Geometry: final body of the model. Coordinates: model frame, mm. A direction names the side the tool comes from. Coordinates: 2 decimals unless noted, no trailing zeros. Write each loop counter-clockwise with the first axis right and the second up, starting at its lowest first coordinate (ties: lowest second). Pieces come first, ordered by that corner, then holes.
from build123d import *

# Parameters (mm, degrees)
BOSS_EXTRUDE1_DEPTH = 100
CUT_EXTRUDE1_DEPTH  = 126.95237195067031
FILLET1_R           = 5
BOSS_EXTRUDE2_START = 40.5
BOSS_EXTRUDE2_DEPTH = 40.5
FILLET2_R           = 11
FILLET3_R           = 5
BOSS_EXTRUDE4_DEPTH = 10
FILLET5_R           = 1
FILLET6_R           = 5
SKETCH8_R           = 7.5
CUT_EXTRUDE2_DEPTH  = 131.85870255202755
SKETCH9_R           = 1.2499999999993074
SKETCH9_R_2         = 1.2499999999993041
SKETCH9_R_3         = 1.2499999999993108
CUT_EXTRUDE3_DEPTH  = 131.85870255202755
SKETCH10_R          = 2.999999999999271
SKETCH10_R_2        = 2.9999999999993827
SKETCH10_R_3        = 2.9999999999993676
SKETCH10_R_4        = 2.9999999999984848
CUT_EXTRUDE4_DEPTH  = 5


with BuildPart() as part:
    # Sketch1 → Boss-Extrude1 (new body)
    with BuildSketch(Plane(origin=(0, 0, 0), x_dir=(1, 0, 0), z_dir=(0, 1, 0))):
        Polygon((-29.000000000000004, -50), (-29.000000000000004, 50), (28.999999999999996, 50.00000000000001), (28.999999999999996, -50), (22.5, -50), (22.49999999999999, 20.000000000000004), (-18.000000000000007, 20.000000000000004), (-18.000000000000007, -50), align=None)
    extrude(amount=BOSS_EXTRUDE1_DEPTH)

    # Sketch5 → Cut-Extrude1 (cut, through all)
    with BuildSketch(Plane(origin=(28.999999999999996, 0, 0), x_dir=(0, 0, -1), z_dir=(1, 0, 0))):
        with BuildLine():
            Line((50.00000000000001, 94), (15.000000000000007, 94))
            Line((15.000000000000007, 94), (-15.988977704079698, 68.21854812358211))
            ThreePointArc((-15.988977704079698, 68.21854812358211), (-24.331609312743236, 43.25780632057522), (-5.709440185764556, 24.660684217398867))
            Line((-5.709440185764556, 24.660684217398867), (44.000000000000014, 12.999999999999998))
            Line((44.000000000000014, 12.999999999999998), (50.00000000000001, 12.999999999999998))
            Line((50.00000000000001, 12.999999999999998), (50.00000000000001, 94))
        make_face()
        with BuildLine():
            Line((12.83046096501491, 100), (-19.82633235305885, 72.8309996732418))
            ThreePointArc((-19.82633235305885, 72.8309996732418), (-30.160384185664846, 41.83402304126666), (-6.988314668956372, 18.797956061093338))
            Line((-6.988314668956372, 18.797956061093338), (44, 6.999999999999997))
            Line((44, 6.999999999999997), (49.99999999999999, 6.999999999999992))
            Line((49.99999999999999, 6.999999999999992), (49.99999999999999, 0))
            Line((49.99999999999999, 0), (-50.00000000000001, 0))
            Line((-50.00000000000001, 0), (-50.00000000000001, 100))
            Line((-50.00000000000001, 100), (12.83046096501491, 100))
        make_face()
    extrude(amount=-CUT_EXTRUDE1_DEPTH, mode=Mode.SUBTRACT)

    # Fillet1
    fillet1_edges = [part.edges().sort_by_distance(p)[0] for p in [
        (-23.500000000000004, 94, -15.000000000000007),
        (25.749999999999993, 94, -15.000000000000007),
    ]]
    fillet(fillet1_edges, radius=FILLET1_R)

    # Sketch6 → Boss-Extrude2 (add)
    with BuildSketch(Plane(origin=(-18.000000000000007, 0, 0), x_dir=(1e-16, 0, -1), z_dir=(1, 0, 1e-16)).offset(BOSS_EXTRUDE2_START)):
        with BuildLine():
            Line((19.999999999999996, 12.553251706878484), (-6.988314668956373, 18.79795606109335))
            ThreePointArc((-6.988314668956373, 18.79795606109335), (-27.865951255157718, 35.417336025463435), (-28.095541398136127, 62.1011661139617))
            Line((-28.095541398136127, 62.1011661139617), (-22.657694675916233, 59.56545654351749))
            ThreePointArc((-22.657694675916233, 59.56545654351749), (-22.489094420401646, 38.08026409887772), (-5.709440185764564, 24.66068421739888))
            Line((-5.709440185764564, 24.66068421739888), (19.999999999999993, 18.62984455611945))
            Line((19.999999999999993, 18.62984455611945), (19.999999999999996, 12.553251706878484))
        make_face()
    extrude(amount=-BOSS_EXTRUDE2_DEPTH)

    # Fillet2
    fillet2_edges = [part.edges().sort_by_distance(p)[0] for p in [
        (25.749999999999993, 100, -12.83046096501491),
        (-23.500000000000004, 100, -12.83046096501491),
    ]]
    fillet(fillet2_edges, radius=FILLET2_R)

    # Fillet3
    fillet3_edges = [part.edges().sort_by_distance(p)[0] for p in [
        (22.49999999999999, 60.8333113287396, 25.376618037026184),
        (-18.00000000000001, 60.8333113287396, 25.37661803702618),
        (22.49999999999999, 97, -20.000000000000004),
        (-18.000000000000007, 97, -20.000000000000004),
    ]]
    fillet(fillet3_edges, radius=FILLET3_R)

    # Sketch7 → Boss-Extrude4 (add)
    with BuildSketch(Plane(origin=(28.999999999999996, 0, 0), x_dir=(0, 0, -1), z_dir=(1, 0, 0))):
        with BuildLine():
            Line((50.00000000000001, 100), (16.807949195820918, 100))
            ThreePointArc((16.807949195820918, 100), (13.067479500591284, 99.34450996708247), (9.772799006025844, 97.45616117437613))
            Line((9.772799006025844, 97.45616117437613), (-19.82633235305885, 72.8309996732418))
            ThreePointArc((-19.82633235305885, 72.8309996732418), (-30.160384185664846, 41.83402304126666), (-6.9883146689563755, 18.797956061093355))
            Line((-6.9883146689563755, 18.797956061093355), (44, 6.999999999999997))
            Line((44, 6.999999999999997), (49.99999999999999, 6.999999999999992))
            Line((49.99999999999999, 6.999999999999992), (50.00000000000001, 100))
        make_face()
    extrude(amount=BOSS_EXTRUDE4_DEPTH)

    # Fillet5
    fillet5_edges = [part.edges().sort_by_distance(p)[0] for p in [
        (22.49999999999999, 99.00083975111619, -12.227206431541916),
        (-18.000000000000007, 85.14358042380897, 5.026766673516516),
        (22.499999999999993, 69.84794587448418, 22.942605623916762),
        (2.2499999999999893, 62.10116611396171, 28.095541398136127),
        (-18.000000000000007, 99.00083975111619, -12.227206431541916),
        (2.2499999999999893, 100, -20.000000000000004),
        (21.042619780265184, 63.42008867833863, 27.44195770208064),
        (-16.542619780265202, 63.42008867833864, 27.441957702080636),
        (20.324911858881205, 100, -19.12551487569155),
        (22.415270684599754, 99.96382489332538, -15.916577372895661),
        (-17.91527069193968, 99.96382489235059, -15.916577374222168),
        (-15.824911858881226, 100, -19.125514875691554),
        (-18.000000000000004, 69.84794587448418, 22.942605623916755),
        (22.49999999999999, 85.14358042380897, 5.026766673516505),
    ]]
    fillet(fillet5_edges, radius=FILLET5_R)

    # Fillet6
    fillet6_edges = [part.edges().sort_by_distance(p)[0] for p in [
        (39, 12.898978030546676, -18.50584266552181),
        (39, 41.834023041266654, 30.16038418566485),
        (39, 85.14358042380897, 5.026766673516503),
        (39, 99.34450996708247, -13.067479500591286),
        (39, 100, -33.40397459791046),
    ]]
    fillet(fillet6_edges, radius=FILLET6_R)

    # Sketch8 → Cut-Extrude2 (cut, through all)
    with BuildSketch(Plane(origin=(39, 0, 0), x_dir=(0, 0, -1), z_dir=(1, 0, 0))):
        with Locations((-6.94e-15, 49)):
            Circle(SKETCH8_R)
    extrude(amount=-CUT_EXTRUDE2_DEPTH, mode=Mode.SUBTRACT)

    # Sketch9 → Cut-Extrude3 (cut, through all)
    with BuildSketch(Plane(origin=(39, 0, 0), x_dir=(0, 0, -1), z_dir=(1, 0, 0))):
        with Locations((40.00000000000071, 19.744580488536943)):
            Circle(SKETCH9_R)
        with Locations((6.9389e-13, 29.000000000001137)):
            Circle(SKETCH9_R_2)
        with Locations((-19.999999999998934, 49.000000000000405)):
            Circle(SKETCH9_R_2)
        with Locations((16.807949195821617, 89.00000000000007)):
            Circle(SKETCH9_R_3)
    extrude(amount=-CUT_EXTRUDE3_DEPTH, mode=Mode.SUBTRACT)

    # Sketch10 → Cut-Extrude4 (cut)
    with BuildSketch(Plane(origin=(39, 0, 0), x_dir=(0, 0, -1), z_dir=(1, 0, 0))):
        with Locations((16.807949195821624, 89.00000000000007)):
            Circle(SKETCH10_R)
        with Locations((-19.999999999998906, 49.000000000000405)):
            Circle(SKETCH10_R_2)
        with Locations((-1.388e-14, 29.000000000001066)):
            Circle(SKETCH10_R_3)
        with Locations((40.000000000000725, 19.744580488536943)):
            Circle(SKETCH10_R_4)
    extrude(amount=-CUT_EXTRUDE4_DEPTH, mode=Mode.SUBTRACT)


solid = part.part
Item 1: Set-up query: faces 5 (the flat face through (0, 13, -47)), 6 (the cylindrical face through (-16.57, 61.86, 24.03)), 7 (the cylindrical face through (36.53, 91.53, -18.42)). Return all of +Z, -Z, +X, -X, +Y, -Y with unobstructed straight access to the full face (end or side cutting, diameter ignored); none if empty.
Derived:
face 5: -Z, -X
face 6: -Z, +Y
face 7: +X
Item 2: Material intervals for probe 1 along X at (y, z) = (78, 6.5); probe 2 along Z at (x, y) = (31.5, 48); probe 3 along X at (y, z) = (50.5, 23), sorted ascending.
Derived:
probe 1: x = -29 to -18, 22.5 to 38.98
probe 2: z = -50 to -7.43, 7.43 to 19.25, 20.75 to 30.98
probe 3: x = 29 to 39
Item 3: Section B-B, the plane y = 49. Output: boundary loops of the cut face in (x, z).
Derived:
outline: (-29, 25) - (29, 25) - (29, 21.25) - (34, 21.25) - (34, 23) - (39, 23) - (39, 26) arc R5 ccw to (34, 31) - (-29, 31) - close; (29, -50) - (39, -50) - (39, -7.5) - (29, -7.5) - close; (29, 7.5) - (39, 7.5) - (39, 17) - (34, 17) - (34, 18.75) - (29, 18.75) - close
Item 4: Pull-direction query (Y, two-part tool) for faces 1 (the cylindrical face through (-18.285, 84.74, 5.042)), 2 (the flat face through (34, 18, -40)), 3 (the flat face through (2.06, 12.98, -18.15)), 4 (the cylindrical face through (-23.4, 93.7, -15.1)); classes: released by +Y, released by -Y, zero draft, split by the parting line, or undercut.
Derived:
face 1: released by +Y
face 2: undercut
face 3: released by -Y
face 4: undercut
Item 5: Pin query (flat end, axial travel): pin 1 (5 mm diameter, centred on y = 49, z = 20, fed in from +X); pin 2 (4 mm diameter, centred on x = 12.5, z = 8, fed in from +Y); pin 3 (10 mm diameter, centred on x = -21.5, y = 21, fed in from +Z). Return the tip coordinate at first contact, or that it passes through.
Derived:
pin 1: stops at x = 34
pin 2: stops at y = 26.09
pin 3: stops at z = 20.78
Item 6: Section C-C, the plane z = 0. State how many separate pieces and enclosed holes the cut face has, plus the area to 3 significant figures.
Derived:
separate pieces: 4
enclosed holes: 0
area: 1,010 mm2
Item 7: Section A-A, the plane x = -1. Output: boundary loops of the cut face in (y, z), plus the area to 3 significant figures.
Derived:
outline: (7, -50) - (13, -50) - (13, -44) - (24.66, 5.71) arc R25 cw to (59.57, 22.66) - (61.67, 27.17) arc R1 ccw to (61.16, 28.52) arc R31 ccw to (18.8, 6.99) - (7, -44) - close; (94, -50) - (100, -50) - (100, -21) arc R1 ccw to (99, -20) - (94, -20) - close
area: 820 mm2
